Source: CAD feature listing. Evaluate the final solid. Frame: model axes, mm. Coordinates: 2 decimals unless noted, no trailing zeros. Loops run counter-clockwise (first coordinate to the right, second up) from the corner with the lowest first, then second, coordinate; pieces in that order, holes last.
Item 1: Section query A-A, the plane z = 11. Return the cut outline in (x, y), then the cut area to 3 significant figures.
Item 2: Section query C-C, the plane y = 6. Return the cut outline in (x, z), then the cut area to 3 significant figures.
Item 3: Section query B-B, the plane z = 12.6. Return the cut outline in (x, y).
Item 4: Line query: probe 1 along X at (y, z) = (4.75, 11.75); probe 2 along X at (y, z) = (11, 11.8); probe 3 along X at (y, z) = (1, 11.3). Output: solid intervals per line, ascending.
Item 5: Section query D-D, the plane z = 13.9. Return the cut outline in (x, y), then the cut area to 3 significant figures.
Item 6: Pin query (flat end, axial travel): pin 1 Ø6 at (x, y) = (-1.5, 2) entering from -Z; pin 2 Ø2 at (x, z) = (6, 13.5) entering from -Y; pin 3 Ø2 at (x, y) = (2.5, 7) entering from -Z; pin 4 Ø3.5 at (x, y) = (1.5, 6) entering from +Z. Return the tip coordinate at first contact, or that it passes through.
Solid Edge part; units mm, degrees
sketch "Sketch1" plane through (0, 0, 0) normal (0, -1, 0) x (1, 0, 0)
  circle A0 centre (-5.6109, 12.3912) radius 1.05
  circle A1 centre (12.0891, 12.3912) radius 1.05
  line L0 (-3.9954, 13.3912) -> (10.4735, 13.3912)
  line L1 (10.4735, 11.3912) -> (-3.9954, 11.3912)
  arc A2 (-3.9954, 11.3912) -> (-3.9954, 13.3912) centre (-5.6109, 12.3912) cw
  arc A3 (10.4735, 13.3912) -> (10.4735, 11.3912) centre (12.0891, 12.3912) cw
extrude "Protrusion1" add sketch "Sketch1" against normal blind 11.5
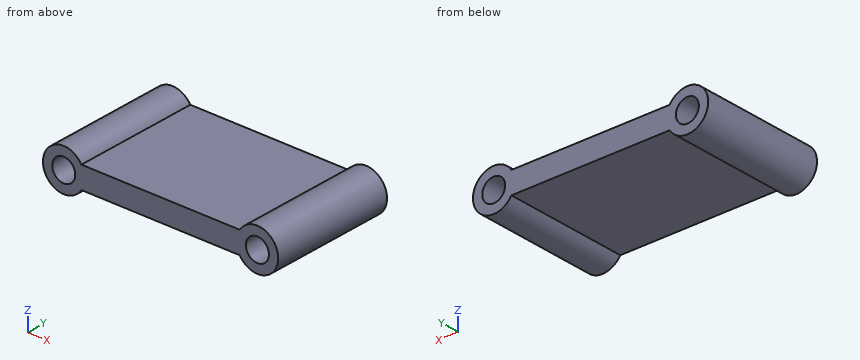
Verdict:
1. outline: (-6.9, 0) - (-4.32, 0) - (-4.32, 11.5) - (-6.9, 11.5) - close; (10.8, 0) - (13.38, 0) - (13.38, 11.5) - (10.8, 11.5) - close
1. area: 59.5 mm2
2. outline: (-4, 11.39) - (10.47, 11.39) arc R1.9 ccw (long way) to (10.47, 13.39) - (-4, 13.39) arc R1.9 ccw (long way) to start; hole circle Ø2.1 at (-5.61, 12.39); hole circle Ø2.1 at (12.09, 12.39)
2. area: 43.9 mm2
3. outline: (-7.5, 0) - (-6.64, 0) - (-6.64, 11.5) - (-7.5, 11.5) - close; (-4.58, 0) - (11.06, 0) - (11.06, 11.5) - (-4.58, 11.5) - close; (13.12, 0) - (13.98, 0) - (13.98, 11.5) - (13.12, 11.5) - close
4. probe 1: x = -7.4 to -6.44, -4.78 to 11.26, 12.92 to 13.88
4. probe 2: x = -7.42 to -6.48, -4.74 to 11.22, 12.96 to 13.89
4. probe 3: x = -7.17 to -4.06, 10.53 to 13.64
5. outline: (-6.77, 0) - (-4.46, 0) - (-4.46, 11.5) - (-6.77, 11.5) - close; (10.93, 0) - (13.24, 0) - (13.24, 11.5) - (10.93, 11.5) - close
5. area: 53.1 mm2
6. pin 1: stops at z = 10.85
6. pin 2: stops at y = 0
6. pin 3: stops at z = 11.39
6. pin 4: stops at z = 13.39
